```python
from build123d import *

# Parameters (mm, degrees)
SKETCH1_R           = 2.5
BOSS_EXTRUDE1_DEPTH = 69
FILLET1_R           = 1
FILLET2_R           = 0.5
FILLET3_R           = 0.5
FILLET4_R           = 0.5
FILLET5_R           = 0.5


with BuildPart() as part:
    # Sketch1 → Boss-Extrude1 (new body)
    with BuildSketch(Plane.XY):
        Polygon((13.2, 0), (13.2, 1.8), (15.45, 1.8), (15.45, 3.6), (12.95, 6.1), (7.05, 6.1), (4.55, 3.6), (4.55, 1.8), (6.8, 1.8), (6.8, 0), (0, 0), (0, 6.8), (1.8, 6.8), (1.8, 4.55), (3.6, 4.55), (6.1, 7.05), (6.1, 12.95), (3.6, 15.45), (1.8, 15.45), (1.8, 13.2), (0, 13.2), (0, 20), (6.8, 20), (6.8, 18.2), (4.55, 18.2), (4.55, 16.4), (7.05, 13.9), (12.95, 13.9), (15.45, 16.4), (15.45, 18.2), (13.2, 18.2), (13.2, 20), (20, 20), (20, 13.2), (18.2, 13.2), (18.2, 15.45), (16.4, 15.45), (13.9, 12.95), (13.9, 7.05), (16.4, 4.55), (18.2, 4.55), (18.2, 6.8), (20, 6.8), (20, 0), align=None)
        with Locations((10, 10)):
            Circle(SKETCH1_R, mode=Mode.SUBTRACT)
    extrude(amount=BOSS_EXTRUDE1_DEPTH)

    # Fillet1
    fillet1_edges = [part.edges().sort_by_distance(p)[0] for p in [
        (0, 0, 34.5),
        (0, 20, 34.5),
        (20, 20, 34.5),
        (20, 0, 34.5),
    ]]
    fillet(fillet1_edges, radius=FILLET1_R)

    # Fillet2
    fillet2_edges = [part.edges().sort_by_distance(p)[0] for p in [
        (4.55, 18.2, 34.5),
        (4.55, 16.4, 34.5),
        (7.05, 13.9, 34.5),
        (12.95, 13.9, 34.5),
        (15.45, 16.4, 34.5),
        (15.45, 18.2, 34.5),
    ]]
    fillet(fillet2_edges, radius=FILLET2_R)

    # Fillet3
    fillet3_edges = [part.edges().sort_by_distance(p)[0] for p in [
        (18.2, 15.45, 34.5),
        (16.4, 15.45, 34.5),
        (13.9, 12.95, 34.5),
        (13.9, 7.05, 34.5),
        (16.4, 4.55, 34.5),
        (18.2, 4.55, 34.5),
    ]]
    fillet(fillet3_edges, radius=FILLET3_R)

    # Fillet4
    fillet4_edges = [part.edges().sort_by_distance(p)[0] for p in [
        (1.8, 4.55, 34.5),
        (3.6, 4.55, 34.5),
        (6.1, 7.05, 34.5),
        (6.1, 12.95, 34.5),
        (3.6, 15.45, 34.5),
        (1.8, 15.45, 34.5),
    ]]
    fillet(fillet4_edges, radius=FILLET4_R)

    # Fillet5
    fillet5_edges = [part.edges().sort_by_distance(p)[0] for p in [
        (15.45, 1.8, 34.5),
        (15.45, 3.6, 34.5),
        (12.95, 6.1, 34.5),
        (7.05, 6.1, 34.5),
        (4.55, 3.6, 34.5),
        (4.55, 1.8, 34.5),
    ]]
    fillet(fillet5_edges, radius=FILLET5_R)


solid = part.part
```
For this review, take the finished solid that the model builds, in its own axes (mm). A direction names the side the tool comes from. Give positions to 0.01 mm unless a question says otherwise; leave off trailing zeros. Loops run counter-clockwise (first coordinate to the right, second up) from the corner with the lowest first, then second, coordinate; pieces in that order, holes last. Notation, with made-up numbers: M 29,11 L 46,11 A13 cw 46,16 Z; hole C 89,29 d7. An arc over 180 degrees is marked long. One line per item, written item: value. Start each with the question number.
Q1. For L1, parallel to Y at x = 2.5, z = 25.5; L2, parallel to X at y = 18.75, z = 35.5, list the stretches that pass through material, from the lowest coordinate up.
Q2. Machinability: for faces 1 (the face through (10, 13.9, 34)), 2 (the face through (19, 13.2, 34)), 3 (the face through (1, 6.8, 34)), 4 (the face through (14, 18.2, 34)), 5 (the face through (13.2, 1, 34)), which of the approach directions +Z, -Z, +X, -X, +Y, -Y give a long, thin tool a straight path to every point of the face, cutting with its end or side? Answer none if there is none.
Q3. Draft analysis for pull direction Y (two halves, no side actions). For faces 6 (the face through (16, 20, 34)), 7 (the face through (19, 6.8, 34)), 8 (the face through (0, 16, 34)), state which applies: released by +Y, released by -Y, zero draft, split by the parting line, or undercut.
Q4. Add section A-A (x = 10). Give the boundary of the cut face in (y, z), and give its area (3 significant figures).
Q5. Clearance check with a flat-ended pin moving along its axis: pin 1 Ø2 at (y, z) = (0.5, 50.5) entering from +X. State where the tip first meets the part, or that it passes through.
Reply:
1. L1: 0 to 4.55, 15.45 to 20
1. L2: 0 to 6.8, 13.2 to 20
2. face 1: +Z, -Z, +Y
2. face 2: +Z, -Z, +X
2. face 3: +Z, -Z, -X
2. face 4: +Z, -Z
2. face 5: +Z, -Z, -Y
3. face 6: released by +Y
3. face 7: undercut
3. face 8: zero draft
4. outline: M 6.1,0 L 7.5,0 L 7.5,69 L 6.1,69 Z; M 12.5,0 L 13.9,0 L 13.9,69 L 12.5,69 Z
4. area: 193 mm²
5. pin 1: x = 20
